For this review, use the dimensioned drawing (mm, ordinates from the lowest corner) and the shaded views. Round coordinates to 2 decimals unless told otherwise and drop trailing zeros. Loops run counter-clockwise (first coordinate to the right, second up) from the corner with the lowest first, then second, coordinate; pieces in that order, holes last.
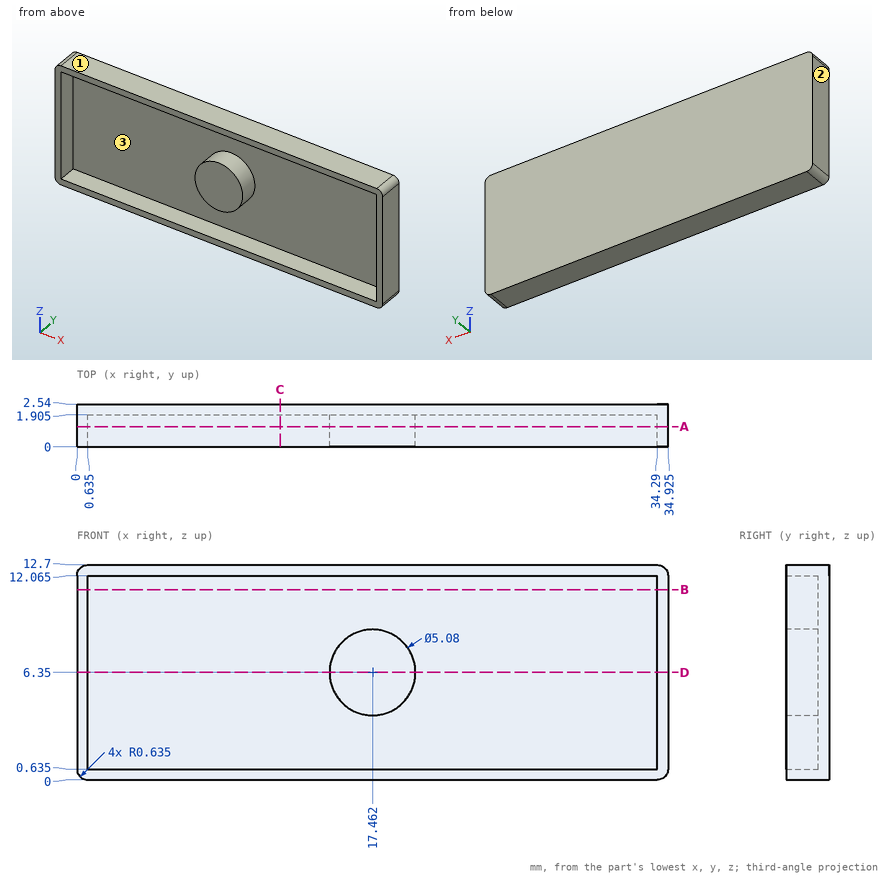
(1) The part is to be moulded in two halves that separate along X. For the marked faces 1, 2 and 3, say which applies: pulls with the +X half, pulls with the -X half, needs draft (parallel to the pull), parting line crosses it, or undercut.
(2) Add section B-B (z = 11.25). Give the boundary of the cut face in (x, y) (1 decimal).
(3) Insertion check: pin 1 Ø1 at (x, z) = (17.5, 11.5) entering from -Y (1 decimal); pin 2 Ø1 at (y, z) = (1.5, 4) entering from -X. Each pin has a flat end and moves straight along its axis. Give the tip position at first contact, or say it passes through.
(4) Add section C-C (x = 12). Give the boundary of the cut face in (y, z) (1 decimal).
(5) Add section A-A (y = 1.2). Give the number of separate pieces and of enclosed holes in the cut face.
(6) For L1, parallel to X at y = 1.8, z = 6.5 (1 decimal); L2, parallel to X at y = 1.7, z = 11.5 (1 decimal); L3, parallel to Z at x = 1, y = 0.3 (1 decimal), list the stretches that pass through material, from the lowest coordinate up.
(7) Add section D-D (z = 6.35). Give the boundary of the cut face in (x, y) (1 decimal).
Outcome:
1. face 1: needs draft
1. face 2: pulls with the -X half
1. face 3: undercut
2. outline: (0, 0) - (0.6, 0) - (0.6, 1.9) - (34.3, 1.9) - (34.3, 0) - (34.9, 0) - (34.9, 2.5) - (0, 2.5) - close
3. pin 1: stops at y = 1.9
3. pin 2: stops at x = 0
4. outline: (0, 0) - (2.5, 0) - (2.5, 12.7) - (0, 12.7) - (0, 12.1) - (1.9, 12.1) - (1.9, 0.6) - (0, 0.6) - close
5. separate pieces: 2
5. enclosed holes: 1
6. L1: x = 0 to 0.6, 14.9 to 20, 34.3 to 34.9
6. L2: x = 0 to 0.6, 34.3 to 34.9
6. L3: z = 0 to 0.6, 12.1 to 12.7
7. outline: (0, 0) - (0.6, 0) - (0.6, 1.9) - (14.9, 1.9) - (14.9, 0) - (20, 0) - (20, 1.9) - (34.3, 1.9) - (34.3, 0) - (34.9, 0) - (34.9, 2.5) - (0, 2.5) - close
